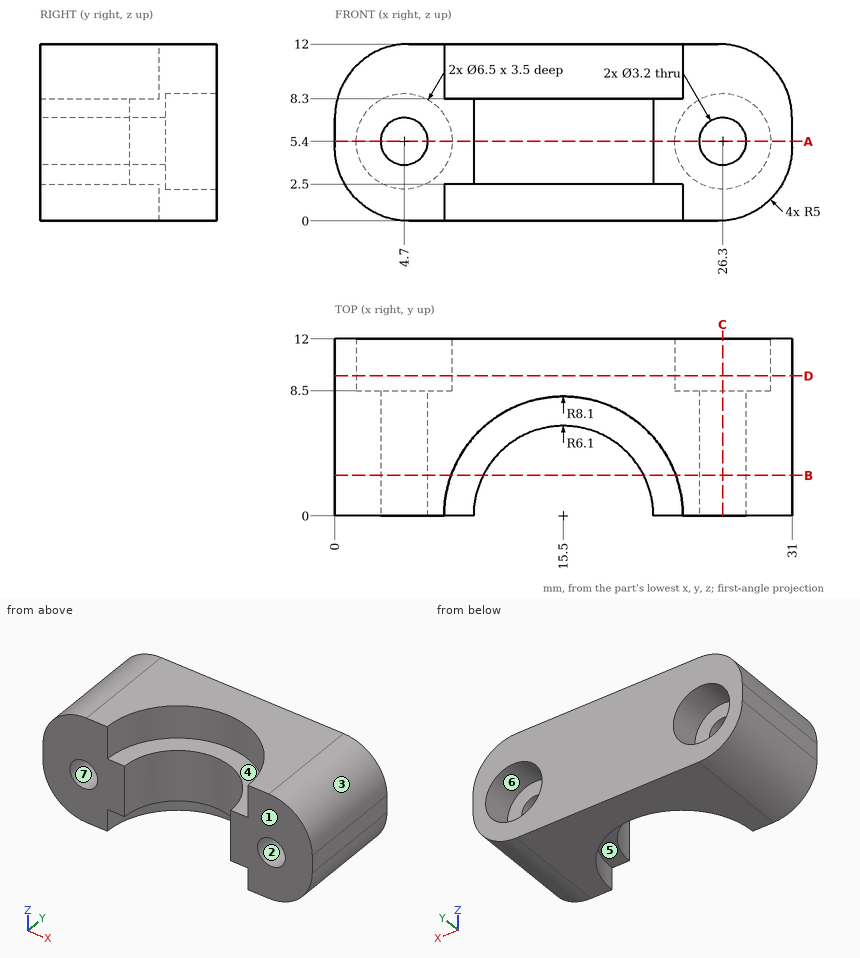
Source: three-view drawing plus pictorial views. Frame: mm from the lowest corner of the part. A direction names the side the tool comes from. Give positions to 0.01 mm unless a question says otherwise; leave off trailing zeros. Order: outer loops, then holes, each group sorted by start corner. A loop starts at its lowest first (then second) coordinate and runs counter-clockwise, first axis right, second up. Notation, with made-up numbers: (-28, 61.25) -> (-4, 61.25) arc R21 cw to (-4, 86.25) -> close; hole circle Ø8 at (12.5, 12.5). An arc over 180 degrees is marked (long way). Use a Markdown table: item, result.
Q1. Section D-D (y = 9.5). Return the cut outline in (x, z), and give its area (3 significant figures).
A:
| item | result |
|---|---|
| outline | (0, 5) arc R5 ccw to (5, 0) -> (26, 0) arc R5 ccw to (31, 5) -> (31, 7) arc R5 ccw to (26, 12) -> (5, 12) arc R5 ccw to (0, 7) -> close; hole circle Ø6.5 at (4.7, 5.4); hole circle Ø6.5 at (26.3, 5.4) |
| area | 284 mm^2 |
Q2. Section B-B (y = 2.75). Return the cut outline in (x, z).
A:
| item | result |
|---|---|
| outline | (0, 5) arc R5 ccw to (5, 0) -> (7.88, 0) -> (7.88, 2.5) -> (10.06, 2.5) -> (10.06, 8.3) -> (7.88, 8.3) -> (7.88, 12) -> (5, 12) arc R5 ccw to (0, 7) -> close; (20.94, 2.5) -> (23.12, 2.5) -> (23.12, 0) -> (26, 0) arc R5 ccw to (31, 5) -> (31, 7) arc R5 ccw to (26, 12) -> (23.12, 12) -> (23.12, 8.3) -> (20.94, 8.3) -> close; hole circle Ø3.2 at (4.7, 5.4); hole circle Ø3.2 at (26.3, 5.4) |
Q3. Pull-direction query (X, two-part tool) for the marked faces 1, 2 and 3; classes: +X half, -X half, draft (parallel to the pull), parting line (faces both ways), or undercut.
A:
| item | result |
|---|---|
| face 1 | draft |
| face 2 | undercut |
| face 3 | +X half |
Q4. Access query for the marked faces 4, 5, 6 and 7. Directions: +Z, -Z, +X, -X, +Y, -Y. A direction counts if a zero-diameter tool reaches every point of the face in a straight line with its end or side. Return the directions, or none.
A:
| item | result |
|---|---|
| face 4 | +Z, -Y |
| face 5 | -Z, -Y |
| face 6 | +Y |
| face 7 | +Y, -Y |
Q5. Section A-A (z = 5.4). Return the cut outline in (x, y).
A:
| item | result |
|---|---|
| outline | (0, 0) -> (3.1, 0) -> (3.1, 8.5) -> (1.45, 8.5) -> (1.45, 12) -> (0, 12) -> close; (6.3, 0) -> (9.4, 0) arc R6.1 cw to (21.6, 0) -> (24.7, 0) -> (24.7, 8.5) -> (23.05, 8.5) -> (23.05, 12) -> (7.95, 12) -> (7.95, 8.5) -> (6.3, 8.5) -> close; (27.9, 0) -> (31, 0) -> (31, 12) -> (29.55, 12) -> (29.55, 8.5) -> (27.9, 8.5) -> close |
Q6. First-contact query: P1, Ø2, axis at x = 26.5, z = 4, coming from the +Y side; P2, Ø5, axis at y = 5.5, z = 10, coming from the +X side; P3, Ø1, axis at x = 27, y = 3.5, coming from the +Z side. Flat tips, straight axial feed; report the tip coordinate or a pass-through.
A:
| item | result |
|---|---|
| P1 | y = 8.5 |
| P2 | x = 30.97 |
| P3 | z = 11.97 |
Q7. Section C-C (x = 26.3). Return the cut outline in (y, z), and give its area (3 significant figures).
A:
| item | result |
|---|---|
| outline | (0, 0.01) -> (12, 0.01) -> (12, 2.15) -> (8.5, 2.15) -> (8.5, 3.8) -> (0, 3.8) -> close; (0, 7) -> (8.5, 7) -> (8.5, 8.65) -> (12, 8.65) -> (12, 11.99) -> (0, 11.99) -> close |
| area | 93.8 mm^2 |
Q8. Material intervals for line 1 (X direction, y = 9.5, z = 4.5); line 2 (Z direction, x = 8, y = 1.75); line 3 (X direction, y = 4.75, z = 9), sorted ascending. Write a range as [from, to].
A:
| item | result |
|---|---|
| line 1 | [0.03, 1.58], [7.82, 23.18], [29.42, 30.97] |
| line 2 | [2.5, 8.3] |
| line 3 | [0.42, 8.94], [22.06, 30.58] |
